```python
from build123d import *

# Parameters (mm, degrees)
BOSS_EXTRUDE1_DEPTH = 95.6564
SKETCH2_W           = 92.2655
SKETCH2_H           = 16.129
SKETCH2_R           = 1.27
BOSS_EXTRUDE2_DEPTH = 4.1148


with BuildPart() as part:
    # Sketch1 → Boss-Extrude1 (new body)
    with BuildSketch(Plane.XY):
        Polygon((-28.0289, 0), (28.0289, 0), (28.0289, 1.5494), (23.9903, 1.5494), (23.9903, 24.384), (-28.0289, 24.384), align=None)
    extrude(amount=BOSS_EXTRUDE1_DEPTH)

    # Sketch2 → Boss-Extrude2 (add)
    with BuildSketch(Plane(origin=(23.9903, 0, 0), x_dir=(0, 0, -1), z_dir=(1, 0, 0))):
        with Locations((-47.39005, 14.1986)):
            Rectangle(SKETCH2_W, SKETCH2_H)
        with Locations((-79.2226, 13.4239)):
            Circle(SKETCH2_R, mode=Mode.SUBTRACT)
        with Locations((-41.1734, 13.4239)):
            Circle(SKETCH2_R, mode=Mode.SUBTRACT)
        with Locations((-15.0368, 13.4239)):
            Circle(SKETCH2_R, mode=Mode.SUBTRACT)
    extrude(amount=BOSS_EXTRUDE2_DEPTH)


solid = part.part
```
For this review, take the finished solid that the model builds, in its own axes (mm). A direction names the side the tool comes from. Round coordinates to 2 decimals unless told otherwise and drop trailing zeros. Loops run counter-clockwise (first coordinate to the right, second up) from the corner with the lowest first, then second, coordinate; pieces in that order, holes last.
(1) We need section B-B (y = 4). Give the boundary of the cut face in (x, z), plus the area to 3 significant figures.
Returned:
outline: (-28.03, 0) - (23.99, 0) - (23.99, 95.66) - (-28.03, 95.66) - close
area: 4,980 mm2
(2) We need section A-A (z = 71.5). Give the boundary of the cut face in (x, y).
Returned:
outline: (-28.03, 0) - (28.03, 0) - (28.03, 1.55) - (23.99, 1.55) - (23.99, 6.13) - (28.11, 6.13) - (28.11, 22.26) - (23.99, 22.26) - (23.99, 24.38) - (-28.03, 24.38) - close
(3) Mouldability with a two-part tool opening along Y and no side actions: class faces 4 (the cylindrical face through (26.019, 13.805, 39.962)), 5 (the flat face through (0, 0, 47)), 6 (the flat face through (0, 12, 0)) as released by +Y, released by -Y, zero draft, split by the parting line, or undercut.
Returned:
face 4: undercut
face 5: released by -Y
face 6: zero draft
(4) Clearance check with flat-ended pins moving along their axes: P1, Ø1.2, axis at x = 27, z = 45, coming from the +Y side; P2, Ø2, axis at y = 13.5, z = 15, coming from the +X side; P3, Ø1.2, axis at x = 26, y = 15.5, coming from the +Z side. State where each tip first meets the part, or that it passes through.
Returned:
P1: stops at y = 22.26
P2: stops at x = 23.99
P3: stops at z = 93.52
(5) Wall thickness on line 1 along X through (y, z) = (4.75, 7.5): over which ranges is the line inside the solid? List them lowest first.
Returned:
line 1: x = -28.03 to 23.99
(6) Tool access review of faces 1 (the flat face through (26, 22.263, 48)), 2 (the flat face through (26, 14, 1.257)), 3 (the cylindrical face through (26.019, 14.683, 15.202)): name each direction out of +Z, -Z, +X, -X, +Y, -Y from which nothing blocks a thin tool from reaching the whole face with its end or side.
Returned:
face 1: +Z, -Z, +X, +Y
face 2: -Z, +X, +Y
face 3: +X
